from build123d import *

# Parameters (mm, degrees)
EXTRUDE_1_DEPTH     = 1.5
SKETCH_2_R          = 1
CUT_EXTRUDE_1_DEPTH = 1.5


with BuildPart() as part:
    # Эскиз1 → Бобышка-Вытянуть1 (new body)
    with BuildSketch(Plane.XY):
        with BuildLine():
            Line((-0.321098845, -11.495516323), (-0.226165274, -8.096841932))
            ThreePointArc((-0.226165274, -8.096841932), (0, 8.1), (0.226165274, -8.096841932))
            Line((0.226165274, -8.096841932), (0.321098845, -11.495516323))
            ThreePointArc((0.321098845, -11.495516323), (1.818971328, -11.355234181), (3.285714286, -11.020620746))
            ThreePointArc((3.285714286, -11.020620746), (3.801783726, -10.659920203), (4, -10.062305899))
            Line((4, -10.062305899), (4, -9.810708435))
            ThreePointArc((4, -9.810708435), (4.255443248, -8.832689141), (4.956521739, -8.104498273))
            ThreePointArc((4.956521739, -8.104498273), (0, 9.5), (-4.956521739, -8.104498273))
            ThreePointArc((-4.956521739, -8.104498273), (-4.255443248, -8.832689141), (-4, -9.810708435))
            Line((-4, -9.810708435), (-4, -10.062305899))
            ThreePointArc((-4, -10.062305899), (-3.801783726, -10.659920203), (-3.285714286, -11.020620746))
            ThreePointArc((-3.285714286, -11.020620746), (-1.818971328, -11.355234181), (-0.321098845, -11.495516323))
        make_face()
    extrude(amount=EXTRUDE_1_DEPTH)

    # Эскиз2 → Вырез-Вытянуть1 (cut)
    with BuildSketch(Plane(origin=(0, 0, 0), x_dir=(-1, 0, 0), z_dir=(0, 0, -1))):
        with Locations((-2.177047903, -9.494628436)):
            Circle(SKETCH_2_R)
        with Locations((2.177047903, -9.494628436)):
            Circle(SKETCH_2_R)
    extrude(amount=-CUT_EXTRUDE_1_DEPTH, mode=Mode.SUBTRACT)


solid = part.part
Verification items for the finished model (mm, model axes). Round coordinates to 2 decimals unless told otherwise and drop trailing zeros. Loops run counter-clockwise (first coordinate to the right, second up) from the corner with the lowest first, then second, coordinate; pieces in that order, holes last. Notation, with made-up numbers: (-30.75, 65) - (-22.75, 65) arc R22 cw to (-22.75, 74) - close; hole circle Ø4 at (0.25, 50). An arc over 180 degrees is marked (long way). Use a Markdown table: item, result. Add a question column.
1. Section check B-B, the plane x = -7. Record the boundary of the cut face in (y, z).
2. Section check A-A, the plane y = 0. Record the boundary of the cut face in (x, z), plus the area to 3 significant figures.
3. Release check for a two-part mould opening along Y. For faces 1 (the face through (3.796, -10.667, 0.74)), 2 (the face through (2.914, -8.819, 0.74)), 3 (the face through (-4.3, -7.2, 1.5)), 4 (the face through (-0.353, 8.092, 0.74)) record: released by +Y, released by -Y, zero draft, split by the parting line, or undercut.
4. Section check D-D, the plane x = 2. Record the boundary of the cut face in (y, z), plus the area to 3 significant figures.
5. Gauge pin test, flat end, axial feed: pin 1 (1.6 mm diameter, centred on x = -2.18, y = -9.49, fed in from -Z). Record the tip position at first contact, or that the pin passes through.
6. Section check C-C, the plane z = 0.35. Record the boundary of the cut face in (x, y).
7. Thickness scan on probe 1 along Y at (x, z) = (1.5, 1.4); probe 2 along Y at (x, z) = (-2.25, 0.65); probe 3 along X at (y, z) = (-0.25, 0.85). Record the ranges inside material, lowest first. Write a range as [from, to].
Checks:
| question | item | result |
|---|---|---|
| 1 | outline | (-6.42, 0) - (-4.08, 0) - (-4.08, 1.5) - (-6.42, 1.5) - close; (4.08, 0) - (6.42, 0) - (6.42, 1.5) - (4.08, 1.5) - close |
| 2 | outline | (-9.5, 0) - (-8.1, 0) - (-8.1, 1.5) - (-9.5, 1.5) - close; (8.1, 0) - (9.5, 0) - (9.5, 1.5) - (8.1, 1.5) - close |
| 2 | area | 4.20 mm^2 |
| 3 | face 1 | released by -Y |
| 3 | face 2 | undercut |
| 3 | face 3 | zero draft |
| 3 | face 4 | undercut |
| 4 | outline | (-11.32, 0) - (-10.48, 0) - (-10.48, 1.5) - (-11.32, 1.5) - close; (-8.51, 0) - (-7.85, 0) - (-7.85, 1.5) - (-8.51, 1.5) - close; (7.85, 0) - (9.29, 0) - (9.29, 1.5) - (7.85, 1.5) - close |
| 4 | area | 4.42 mm^2 |
| 5 | pin 1 | passes through |
| 6 | outline | (-4.96, -8.1) arc R2 cw to (-4, -9.81) - (-4, -10.06) arc R1 ccw to (-3.29, -11.02) arc R11.5 ccw to (-0.32, -11.5) - (-0.23, -8.1) arc R8.1 cw (long way) to (0.23, -8.1) - (0.32, -11.5) arc R11.5 ccw to (3.29, -11.02) arc R1 ccw to (4, -10.06) - (4, -9.81) arc R2 cw to (4.96, -8.1) arc R9.5 ccw (long way) to start; hole circle Ø2 at (-2.18, -9.49); hole circle Ø2 at (2.18, -9.49) |
| 7 | probe 1 | y = [-11.4, -10.23], [-8.76, -7.96], [7.96, 9.38] |
| 7 | probe 2 | y = [-11.28, -10.49], [-8.5, -7.78], [7.78, 9.23] |
| 7 | probe 3 | x = [-9.5, -8.1], [8.1, 9.5] |
